Geometry check sheet. Reference: drawing and pictorial views, mm from the part's lowest x, y, z. Coordinates: 2 decimals unless noted, no trailing zeros. Order: outer loops, then holes, each group sorted by start corner. A loop starts at its lowest first (then second) coordinate and runs counter-clockwise, first axis right, second up. Notation, with made-up numbers: (65.25, 80.25) -> (86.25, 80.25) arc R19 cw to (86.25, 101.25) -> close; hole circle Ø8 at (36, 23.25). An arc over 180 degrees is marked (long way). Use CSV: the item, a comma, the result in double quotes. Start each with the question number.
1) Sectioned sample at C-C on x = 10. Record the boundary of the cut face in (y, z), then the cut area to 3 significant figures.
2) Release check for a two-part mould opening along Y. For the marked faces 1, 2 and 3 record: released by +Y, released by -Y, zero draft, split by the parting line, or undercut.
3) Sectioned sample at A-A on y = 5. Record the boundary of the cut face in (x, z), then the cut area to 3 significant figures.
4) Scan lines: line 1 along Y through (x, z) = (13.5, 5); line 2 along Z through (x, y) = (23.5, 6.25). Record each from-to range of solid material in increasing order.
5) Go/stop test with flat-tipped pins: pin 1 (6 mm diameter, centred on x = 10.5, y = 6.5, fed in from +Z); pin 2 (2 mm diameter, centred on x = 20, z = 3, fed in from -Y); pin 3 (5 mm diameter, centred on x = 22, y = 1, fed in from -Z). Record where each tip stops, or that it passes through.
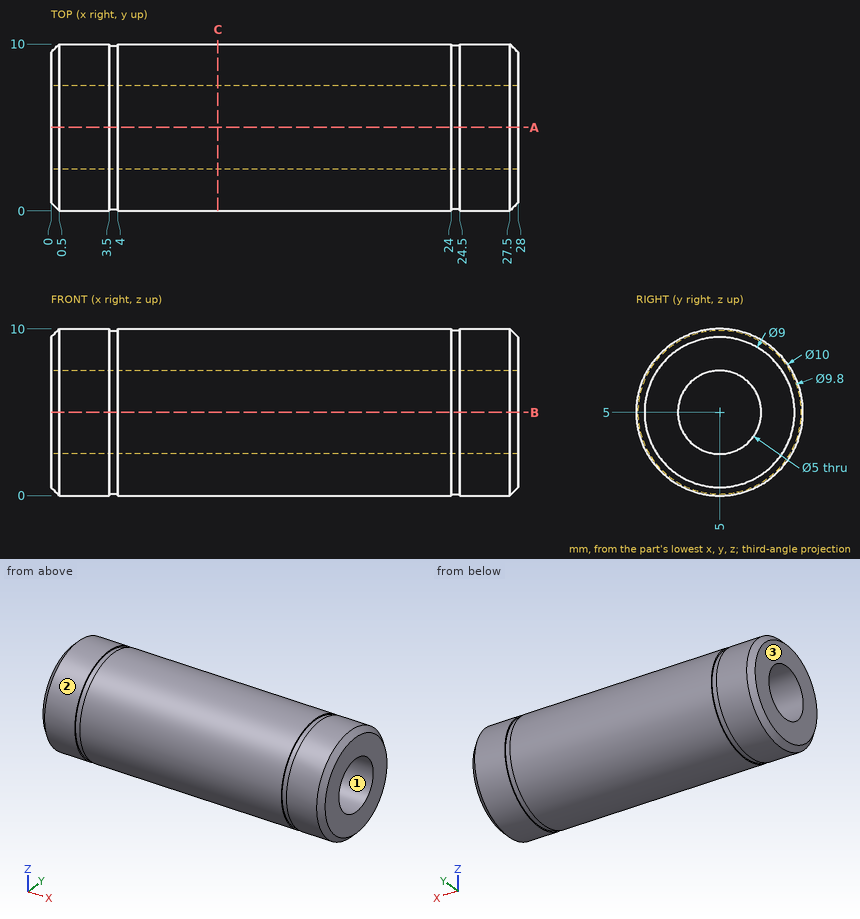
Answers follow:
1,outline,"circle Ø10 at (5, 5); hole circle Ø5 at (5, 5)"
1,area,"58.9 mm²"
2,face 1,"undercut"
2,face 2,"split by the parting line"
2,face 3,"zero draft"
3,outline,"(0, 0.5) -> (0.5, 0) -> (3.5, 0) -> (3.5, 0.1) -> (4, 0.1) -> (4, 0) -> (24, 0) -> (24, 0.1) -> (24.5, 0.1) -> (24.5, 0) -> (27.5, 0) -> (28, 0.5) -> (28, 2.5) -> (0, 2.5) -> close; (0, 7.5) -> (28, 7.5) -> (28, 9.5) -> (27.5, 10) -> (24.5, 10) -> (24.5, 9.9) -> (24, 9.9) -> (24, 10) -> (4, 10) -> (4, 9.9) -> (3.5, 9.9) -> (3.5, 10) -> (0.5, 10) -> (0, 9.5) -> close"
3,area,"139 mm²"
4,line 1,"y = 0 to 2.5, 7.5 to 10"
4,line 2,"z = 0.16 to 2.83, 7.17 to 9.84"
5,pin 1,"stops at z = 10"
5,pin 2,"stops at y = 0.1"
5,pin 3,"stops at z = 0.23"
